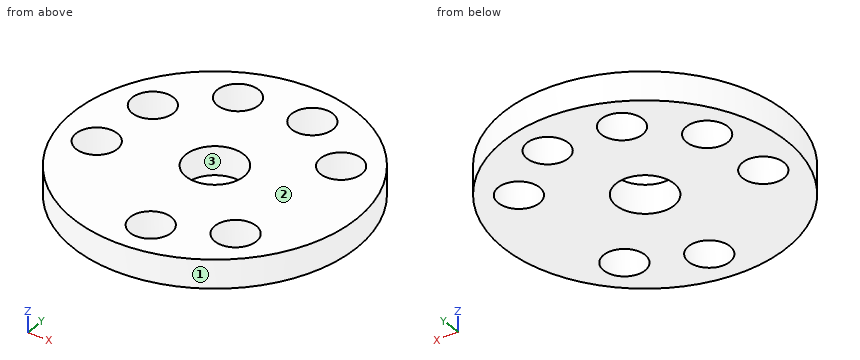
from build123d import *

# Parameters (mm, degrees)
SKETCH8_R           = 49.56483005
BOSS_EXTRUDE3_DEPTH = 10
SKETCH9_R           = 10.176647679
CUT_EXTRUDE3_DEPTH  = 11
SKETCH11_R          = 7.242372995
CUT_EXTRUDE5_DEPTH  = 11
CIRPATTERN2_COUNT   = 9


with BuildPart() as part:
    # Sketch8 → Boss-Extrude3 (new body)
    with BuildSketch(Plane.XY):
        Circle(SKETCH8_R)
    extrude(amount=BOSS_EXTRUDE3_DEPTH)

    # Sketch9 → Cut-Extrude3 (cut, through all)
    with BuildSketch(Plane.XY.offset(10)):
        Circle(SKETCH9_R)
    extrude(amount=-CUT_EXTRUDE3_DEPTH, mode=Mode.SUBTRACT)

    # Sketch11 → Cut-Extrude5 (cut, through all)
    with BuildSketch(Plane.XY.offset(10)):
        with Locations((-14.621394537, 33.273921214)):
            Circle(SKETCH11_R)
    cut_extrude5 = extrude(amount=-CUT_EXTRUDE5_DEPTH, mode=Mode.SUBTRACT)

    # CirPattern2: Cut-Extrude5 ×9 about axis, 2 skipped
    cirpattern2_axis = Axis((0, 0, 0), (0, 0, 1))
    add([cut_extrude5.rotate(cirpattern2_axis, i * 360 / CIRPATTERN2_COUNT) for i in range(1, CIRPATTERN2_COUNT) if i not in (3, 6)], mode=Mode.SUBTRACT)


solid = part.part
Read the model definition and answer for the solid it produces. Units are mm, in the model's axes. Face numbers are marked on the shaded views. Coordinates: 2 decimals unless noted, no trailing zeros. Order: outer loops, then holes, each group sorted by start corner. A loop starts at its lowest first (then second) coordinate and runs counter-clockwise, first axis right, second up. Notation, with made-up numbers: (17, -17.75) -> (46, -17.75) arc R27 ccw to (46, 21.25) -> close; hole circle Ø10 at (82.5, -9). An arc over 180 degrees is marked (long way). Answer as a JSON object with one key per item and string values.
1) Consider line 1 along Y through (x, z) = (0, 3); line 2 along X through (y, z) = (-4, 4.75); line 3 along X through (y, z) = (-7, 8.25). Determine where each line is inside the solid, lowest interval first. Write a range as from..to.
Model answer:
{"line 1": "y = -49.56..-43.12, -29.42..-10.18, 10.18..49.56", "line 2": "x = -49.4..-40.88, -29.73..-9.36, 9.36..49.4", "line 3": "x = -49.07..-42.37, -28.25..-7.39, 7.39..49.07"}
2) Each of these flat-tipped pins is pushed along its axis until it touches: pin 1 (6 mm diameter, centred on y = -35, z = 4, fed in from +X); pin 2 (2 mm diameter, centred on y = 17.5, z = 8, fed in from +X); pin 3 (6 mm diameter, centred on x = -9, z = 2.5, fed in from +Y). Where does it stop, or does it pass through?
Model answer:
{"pin 1": "stops at x = 37.85", "pin 2": "stops at x = 46.74", "pin 3": "stops at y = 49.2"}
3) A cutting plane is placed at C-C, the plane y = 18.5. Determine the outline of the cut face in (x, z).
Model answer:
{"outline": "(-45.98, 0) -> (-39.42, 0) -> (-39.42, 10) -> (-45.98, 10) -> close; (-25.76, 0) -> (23.18, 0) -> (23.18, 10) -> (-25.76, 10) -> close; (37.27, 0) -> (45.98, 0) -> (45.98, 10) -> (37.27, 10) -> close"}
4) A cutting plane is placed at A-A, the plane y = 0. Determine the outline of the cut face in (x, z).
Model answer:
{"outline": "(-49.56, 0) -> (-10.18, 0) -> (-10.18, 10) -> (-49.56, 10) -> close; (10.18, 0) -> (49.56, 0) -> (49.56, 10) -> (10.18, 10) -> close"}
5) A cutting plane is placed at B-B, the plane x = 29.5. Determine the outline of the cut face in (y, z), plus the area to 3 significant figures.
Model answer:
{"outline": "(-39.83, 0) -> (-32.03, 0) -> (-32.03, 10) -> (-39.83, 10) -> close; (-20.5, 0) -> (12.97, 0) -> (12.97, 10) -> (-20.5, 10) -> close; (27.38, 0) -> (39.83, 0) -> (39.83, 10) -> (27.38, 10) -> close", "area": "537 mm²"}
6) A cutting plane is placed at D-D, the plane z = 2.5. State how many separate pieces and enclosed holes the cut face has, plus the area to 3 significant figures.
Model answer:
{"separate pieces": "1", "enclosed holes": "8", "area": "6,240 mm²"}
7) The mould has two halves that part along Y. Classify the marked faces 1, 2 and 3: released by +Y, released by -Y, zero draft, split by the parting line, or undercut.
Model answer:
{"face 1": "split by the parting line", "face 2": "zero draft", "face 3": "undercut"}
